```python
from build123d import *

# Parameters (mm, degrees)
F3_DEPTH     = 0.2
F6_DEPTH     = 0.2
F7_COUNT     = 4
F8_T4_DEPTH  = 1.685841494
F8_S5_R      = 0.5555555556
F8_T6_DEPTH  = 2
F8_T10_DEPTH = 1.685841494
F8_S11_R     = 0.5555555556
F8_T12_DEPTH = 2
F8_T16_DEPTH = 1.685841494
F8_S17_R     = 0.5555555556
F8_T18_DEPTH = 2
F8_T22_DEPTH = 1.685841494
F8_S23_R     = 0.5555555556
F8_T24_DEPTH = 2


# Not quite as in the source:
# - a fillet or chamfer that OpenCascade refuses, or shapes differently, is made with other operations: its cross-section is extruded or revolved along the edge and cut away or added
# - a feature names something its author has since deleted; it is built from what else it names


with BuildPart() as f1:
    # F0 (on Front) → F1 (revolve)
    with BuildSketch(Plane.XZ):
        with BuildLine():
            Line((0, 21.5277777778), (0, 0))
            Line((0, 0), (0.5555555556, 0))
            Line((0.5555555556, 0), (0.5555555556, 19.3055555556))
            Line((0.5555555556, 19.3055555556), (0.2793333296, 21.2847222222))
            ThreePointArc((0.2793333296, 21.2847222222), (0.185137187, 21.4585073218), (0, 21.5277777778))
        make_face()
    revolve(axis=Axis((0, 0, 10.7638888889), (0, 0, 1)))

    # F2 (on Front) → F3 (join, symmetric)
    with BuildSketch(Plane.XZ):
        with BuildLine():
            Line((0, 15.4166666667), (0, 3.4722222222))
            Line((0, 3.4722222222), (1.25, 3.4722222222))
            Line((1.25, 3.4722222222), (1.25, 12.0138888889))
            ThreePointArc((1.25, 12.0138888889), (1.0421485482, 12.2663478223), (0.7291666667, 12.3611111111))
            Line((0.7291666667, 12.3611111111), (0.7291666667, 15.4166666667))
            Line((0.7291666667, 15.4166666667), (0, 15.4166666667))
        make_face()
        Polygon((0, 2.7430555556), (0, 0.9375), (1.2847222222, 0.9375), (1.2847222222, 1.4583333333), (1.9791666667, 1.4583333333), (1.6666666667, 2.7430555556), align=None)
    extrude(amount=F3_DEPTH, both=True)

    # F5 (on face) → F6 (join, symmetric)
    with BuildSketch(Plane(origin=(0, 0, 0), x_dir=(0.7071067812, -0.7071067812, 0), z_dir=(-0.7071067812, -0.7071067812, 0))):
        Polygon((0, 19.3055555556), (0, 18.0555555556), (0.6944444444, 18.0555555556), (0.6944444444, 19.3055555556), (0.612062377, 19.8958333333), (0, 19.8958333333), align=None)
    extrude(amount=F6_DEPTH, both=True)

    # F7: F1 ×4 about axis
    f7_axis = Axis((0, 0, 0), (0, 0, 1))


with BuildPart() as f1_1:
    add(f1.part)
    for i in range(1, F7_COUNT):
        add(f1.part.rotate(f7_axis, i * 360 / F7_COUNT))

    # F8: chamfer of 0.25 on 4 edges, made by hand


with BuildPart() as f8_tool2:
    # F8_s3 → F8_t4 (new body)
    with BuildSketch(Plane.XZ.offset(0.842920747)):
        Polygon((-0.7291666667, 15.1666666667), (-0.4791666667, 15.4166666667), (-0.7291666667, 15.4166666667), align=None)
    extrude(amount=-F8_T4_DEPTH)

    # F8_s5 → F8_t6 (cut, symmetric)
    with BuildSketch(Plane.XY.offset(15.3)):
        Circle(F8_S5_R)
    extrude(amount=F8_T6_DEPTH, both=True, mode=Mode.SUBTRACT)


with BuildPart() as f1_2:
    add(f1_1.part)

    # F8_t1: cut F8_tool2
    add(f8_tool2.part, mode=Mode.SUBTRACT)


with BuildPart() as f8_tool8:
    # F8_s9 → F8_t10 (new body)
    with BuildSketch(Plane.YZ.offset(0.842920747)):
        Polygon((-0.7291666667, 15.1666666667), (-0.4791666667, 15.4166666667), (-0.7291666667, 15.4166666667), align=None)
    extrude(amount=-F8_T10_DEPTH)

    # F8_s11 → F8_t12 (cut, symmetric)
    with BuildSketch(Plane.XY.offset(15.3)):
        Circle(F8_S11_R)
    extrude(amount=F8_T12_DEPTH, both=True, mode=Mode.SUBTRACT)


with BuildPart() as f1_3:
    add(f1_2.part)

    # F8_t7: cut F8_tool8
    add(f8_tool8.part, mode=Mode.SUBTRACT)


with BuildPart() as f8_tool14:
    # F8_s15 → F8_t16 (new body)
    with BuildSketch(Plane.XZ.offset(-0.842920747)):
        Polygon((0.7291666667, 15.1666666667), (0.4791666667, 15.4166666667), (0.7291666667, 15.4166666667), align=None)
    extrude(amount=F8_T16_DEPTH)

    # F8_s17 → F8_t18 (cut, symmetric)
    with BuildSketch(Plane.XY.offset(15.3)):
        Circle(F8_S17_R)
    extrude(amount=F8_T18_DEPTH, both=True, mode=Mode.SUBTRACT)


with BuildPart() as f1_4:
    add(f1_3.part)

    # F8_t13: cut F8_tool14
    add(f8_tool14.part, mode=Mode.SUBTRACT)


with BuildPart() as f8_tool20:
    # F8_s21 → F8_t22 (new body)
    with BuildSketch(Plane.YZ.offset(-0.842920747)):
        Polygon((0.4791666667, 15.4166666667), (0.7291666667, 15.1666666667), (0.7291666667, 15.4166666667), align=None)
    extrude(amount=F8_T22_DEPTH)

    # F8_s23 → F8_t24 (cut, symmetric)
    with BuildSketch(Plane.XY.offset(15.3)):
        Circle(F8_S23_R)
    extrude(amount=F8_T24_DEPTH, both=True, mode=Mode.SUBTRACT)


with BuildPart() as f1_5:
    add(f1_4.part)

    # F8_t19: cut F8_tool20
    add(f8_tool20.part, mode=Mode.SUBTRACT)


solid = f1_5.part
```
Could you check a few things on this model? Use its own coordinates, in mm. A direction names the side the tool comes from. Give positions to 0.01 mm unless a question says otherwise; leave off trailing zeros. Order: outer loops, then holes, each group sorted by start corner. A loop starts at its lowest first (then second) coordinate and runs counter-clockwise, first axis right, second up.
Q1. If I drill on line 1 along Y through (x, z) = (0.9, 11.25); line 2 along Z through (x, y) = (-0.05, 1.45), over which ranges is the centre line in solid material (lowest first)?
Q2. Suppose I cut it at A-A, the plane z = 14.75. Write out the boundary of the cut face in (x, y).
Q3. Suppose I cut it at B-B, the plane z = 4.5. Write out the boundary of the cut face in (x, y).
Q4. I'm going to push a flat-ended pin straight in: P1, Ø0.8, axis at y = 1, z = 12.5, coming from the -X side. Where does the tip first touch, or does it pass through?
Q5. For faces 1 (the flat face through (-0.2, 1, 2)), 2 (the flat face through (0.2, -1, 2)), 3 (the flat face through (-1, -0.2, 2)), which set-ups out of +Z, -Z, +X, -X, +Y, -Y let a thin tool reach every point of the face, with its end or its side?
Solution:
1. line 1: y = -0.2 to 0.2
1. line 2: z = 1.46 to 2.74
2. outline: (-0.73, -0.2) - (-0.52, -0.2) arc R0.56 ccw to (-0.2, -0.52) - (-0.2, -0.73) - (0.2, -0.73) - (0.2, -0.52) arc R0.56 ccw to (0.52, -0.2) - (0.73, -0.2) - (0.73, 0.2) - (0.52, 0.2) arc R0.56 ccw to (0.2, 0.52) - (0.2, 0.73) - (-0.2, 0.73) - (-0.2, 0.52) arc R0.56 ccw to (-0.52, 0.2) - (-0.73, 0.2) - close
3. outline: (-1.25, -0.2) - (-0.52, -0.2) arc R0.56 ccw to (-0.2, -0.52) - (-0.2, -1.25) - (0.2, -1.25) - (0.2, -0.52) arc R0.56 ccw to (0.52, -0.2) - (1.25, -0.2) - (1.25, 0.2) - (0.52, 0.2) arc R0.56 ccw to (0.2, 0.52) - (0.2, 1.25) - (-0.2, 1.25) - (-0.2, 0.52) arc R0.56 ccw to (-0.52, 0.2) - (-1.25, 0.2) - close
4. P1: stops at x = -0.2
5. face 1: +Z, -Z, -X, +Y
5. face 2: +Z, -Z, +X, -Y
5. face 3: +Z, -Z, -X, -Y
